The figure shows three views and two pictorial views of one solid part (mm, origin at its lowest corner). Answer the questions. Coordinates: 2 decimals unless noted, no trailing zeros. Order: outer loops, then holes, each group sorted by start corner. A loop starts at its lowest first (then second) coordinate and runs counter-clockwise, first axis right, second up. Notation, with made-up numbers: M -35.5,50.5 L -13.5,50.5 A7 cw -13.5,63.5 Z; hole C 65.5,-5 d3. An arc over 180 degrees is marked long. Use a Markdown table: item, result.
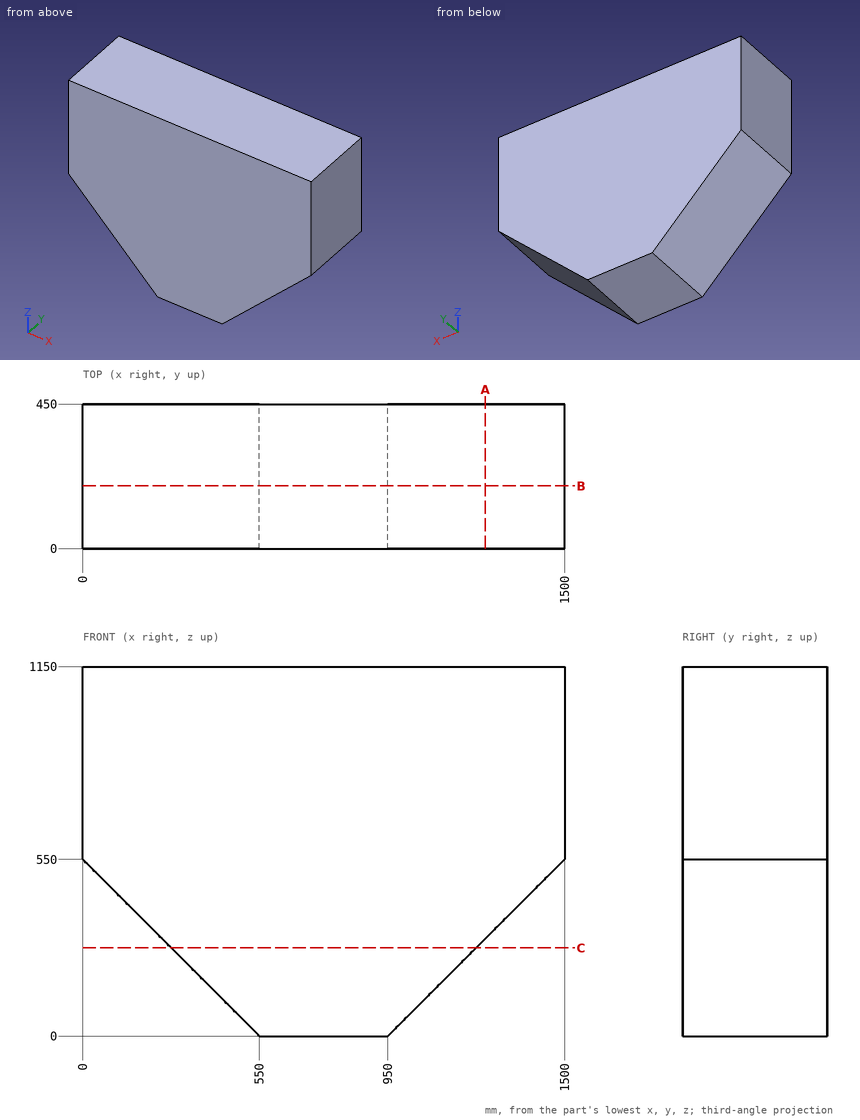
1. Section A-A on x = 1253 is taken. Determine the outline of the cut face in (y, z).
Answers below:
| item | result |
|---|---|
| outline | M 0,303 L 450,303 L 450,1150 L 0,1150 Z |
2. Section C-C on z = 274 is taken. Determine the outline of the cut face in (x, y).
Answers below:
| item | result |
|---|---|
| outline | M 276,0 L 1224,0 L 1224,450 L 276,450 Z |
3. Flat-ended cylindrical pins translate along their axes: P1, Ø2, axis at y = 45.5, z = 405.5, coming from the -X side; P2, Ø8, axis at y = 243.5, z = 358, coming from the +X side; P3, Ø3, axis at y = 108, z = 344.5, coming from the -X side. Find the tip coordinate at first contact, or state that the pin passes through.
Answers below:
| item | result |
|---|---|
| P1 | x = 143.5 |
| P2 | x = 1312 |
| P3 | x = 204 |
4. Find the intervals of material crossed by probe 1 along X at (y, z) = (57.5, 219.5); probe 2 along Z at (x, y) = (440, 72); probe 3 along X at (y, z) = (182.5, 533), in increasing order.
Answers below:
| item | result |
|---|---|
| probe 1 | 330.5 to 1169.5 |
| probe 2 | 110 to 1150 |
| probe 3 | 17 to 1483 |
5. Section B-B on y = 195 is taken. Determine the outline of the cut face in (x, z), then the cut area to 3 significant figures.
Answers below:
| item | result |
|---|---|
| outline | M 0,550 L 550,0 L 950,0 L 1500,550 L 1500,1150 L 0,1150 Z |
| area | 1,420,000 mm² |
